Here's how the part is built. I have some questions about the finished solid (model axes, mm). Face numbers are marked on the shaded views. A direction names the side the tool comes from. Coordinates: 2 decimals unless noted, no trailing zeros. Loops run counter-clockwise (first coordinate to the right, second up) from the corner with the lowest first, then second, coordinate; pieces in that order, holes last. Notation, with made-up numbers: M -12,-18 L 35,-18 A9 ccw 35,-10 Z; hole C -24.75,-14.75 d9. An arc over 180 degrees is marked long. Use one line per item in the form item = value. Start each with the question number.
(1) Imagine slicing it at D-D, the plane z = -38. Please give me the cut outline in (x, y), and give its area (3 significant figures).
(2) Imagine slicing it at C-C, the plane x = -38. Please give me the cut outline in (y, z), and give its area (3 significant figures).
(3) On a 3-axis mill with a long thin cutter (end or side, diameter ignored), from which of +Z, -Z, +X, -X, +Y, -Y can I reach the whole of each face in a straight line? I mean the marked faces 1, 2, 3, 4 and 5. Say none if no direction works.
(4) Will these pins go through, and if not, where does the flat tip stop? P1, Ø4, axis at x = 30.5, z = -19.5, coming from the +Y side; P2, Ø1.5, axis at y = 27.5, z = 10.5, coming from the -X side; P3, Ø8, axis at x = 38, z = 0, coming from the -Y side; P4, Ø6, axis at x = -1.5, y = 17, coming from the -Z side.
(5) Please list where these lines run through material, in increasing order: L1, parallel to X at y = 2.5, z = 0; L2, parallel to Y at x = 34.5, z = -18; L3, parallel to Z at x = 14, y = 30.5.
(6) Thinking about a two-plate mould opening in X: for the marked faces 6, 7 and 8, which applies, +X half, -X half, draft (parallel to the pull), parting line (faces both ways), or undercut?
(7) Imagine slicing it at A-A, the plane x = 0. Please give me the cut outline in (y, z).
(8) Imagine slicing it at B-B, the plane y = 19.5. Please give me the cut outline in (x, z).
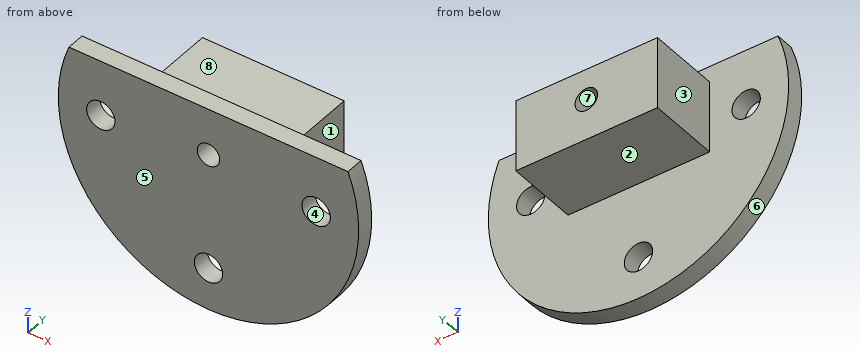
```python
from build123d import *

# Parameters (mm, degrees)
SKETCH1_R           = 5
BOSS_EXTRUDE4_DEPTH = 6.35
SKETCH5_W           = 50
SKETCH5_H           = 25.4
BOSS_EXTRUDE5_DEPTH = 25.4
CUT_EXTRUDE1_START  = -31.75
SKETCH6_R           = 3.96875
CUT_EXTRUDE1_DEPTH  = 31.75


with BuildPart() as part:
    # Sketch1 → Boss-Extrude4 (new body)
    with BuildSketch(Plane(origin=(0, 0, 0), x_dir=(1, 0, 0), z_dir=(0, 1, 0))):
        with BuildLine():
            Line((-49.242854308, -19.599522943), (49.242854308, -19.599522943))
            ThreePointArc((49.242854308, -19.599522943), (0, 53), (-49.242854308, -19.599522943))
        make_face()
        with Locations(Location((-38, 0, 0), (0, 0, 270))):
            Circle(SKETCH1_R, mode=Mode.SUBTRACT)
        with Locations(Location((38, 0, 0), (0, 0, 270))):
            Circle(SKETCH1_R, mode=Mode.SUBTRACT)
        with Locations(Location((0, 38, 0), (0, 0, 270))):
            Circle(SKETCH1_R, mode=Mode.SUBTRACT)
    extrude(amount=BOSS_EXTRUDE4_DEPTH)

    # Sketch5 → Boss-Extrude5 (add)
    with BuildSketch(Plane(origin=(0, 6.35, 0), x_dir=(1, 0, 0), z_dir=(0, 1, 0))):
        with Locations((-0.122917413, -1.3)):
            Rectangle(SKETCH5_W, SKETCH5_H)
    extrude(amount=BOSS_EXTRUDE5_DEPTH)

    # Sketch6 → Cut-Extrude1 (cut)
    with BuildSketch(Plane(origin=(0, 31.75, 0), x_dir=(1, 0, 0), z_dir=(0, 1, 0)).offset(CUT_EXTRUDE1_START)):
        with Locations(Location((0, -3.089464921, 0), (0, 0, 270))):
            Circle(SKETCH6_R)
    extrude(amount=CUT_EXTRUDE1_DEPTH, mode=Mode.SUBTRACT)


solid = part.part
```
Answer:
q1.outline = M -36.95,0 L -5,0 L -5,6.35 L -36.95,6.35 Z; M 5,0 L 36.95,0 L 36.95,6.35 L 5,6.35 Z
q1.area = 406 mm²
q2.outline = M 0,-36.95 L 6.35,-36.95 L 6.35,-5 L 0,-5 Z; M 0,5 L 6.35,5 L 6.35,19.6 L 0,19.6 Z
q2.area = 296 mm²
q3.face_1 = +Z, -Z, +X, +Y
q3.face_2 = -Z, +X, -X, +Y
q3.face_3 = +Z, -Z, -X, +Y
q3.face_4 = +Y, -Y
q3.face_5 = +Z, -Z, +X, -X, -Y
q4.P1 = 6.35
q4.P2 = -25.12
q4.P3 = through
q4.P4 = -11.4
q5.L1 = -53 to -43, -33 to -2.49, 2.49 to 33, 43 to 53
q5.L2 = 0 to 6.35
q5.L3 = -11.4 to 14
q6.face_6 = parting line
q6.face_7 = undercut
q6.face_8 = draft
q7.outline = M 0,-53 L 6.35,-53 L 6.35,-43 L 0,-43 Z; M 0,-33 L 6.35,-33 L 6.35,-11.4 L 31.75,-11.4 L 31.75,-0.88 L 0,-0.88 Z; M 0,7.06 L 31.75,7.06 L 31.75,14 L 6.35,14 L 6.35,19.6 L 0,19.6 Z
q8.outline = M -25.12,-11.4 L 24.88,-11.4 L 24.88,14 L -25.12,14 Z; hole C 0,3.09 d7.94
